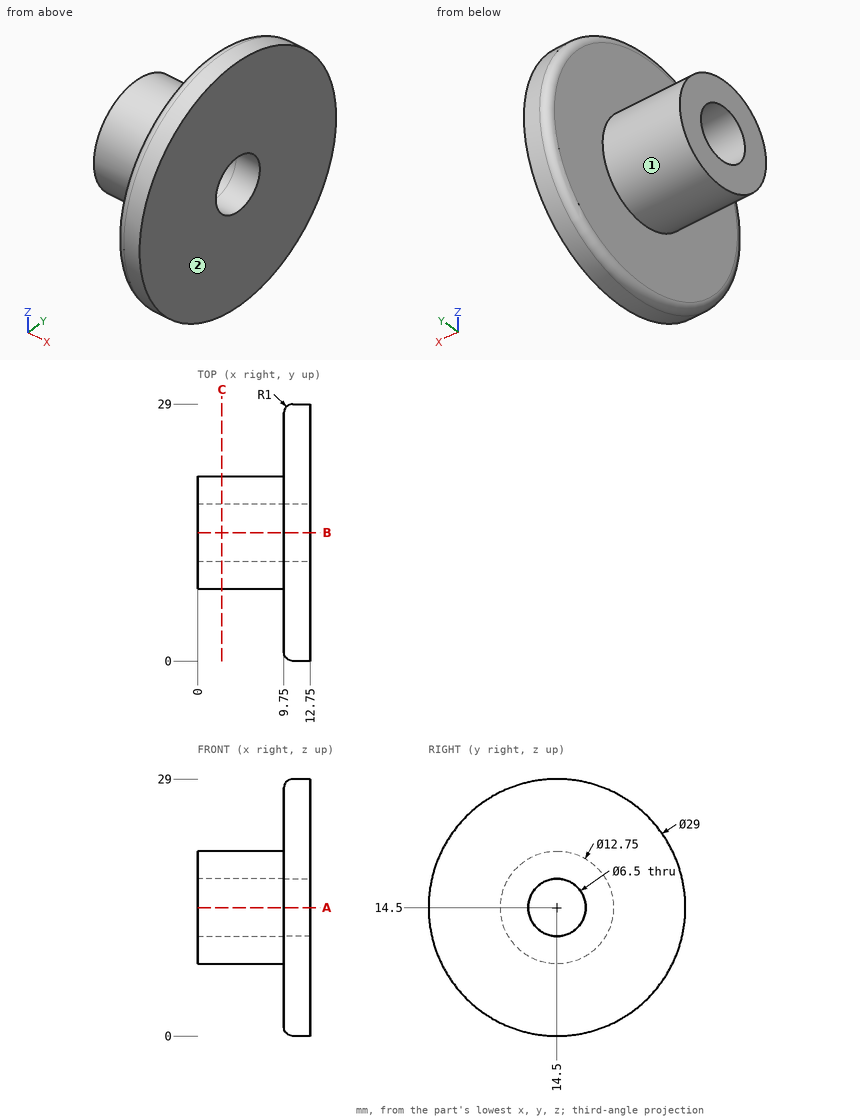
Job drawing, mm, ordinate dimensions from the low corner. One solid piece. A direction names the side the tool comes from. Round coordinates to 2 decimals unless told otherwise and drop trailing zeros. Loops run counter-clockwise (first coordinate to the right, second up) from the corner with the lowest first, then second, coordinate; pieces in that order, holes last. Notation, with made-up numbers: M -34.5,46.25 L 2.5,46.25 A24 cw 2.5,76.25 Z; hole C 54.5,-20.75 d2. An arc over 180 degrees is marked long. One line per question, with ' | ' between items. Start each with the question number.
Item 1: Cut at C-C, the plane x = 2.75. Write the cut outline in (y, z) (3 decimals).
Item 2: Pin check, flat tips, straight feed: pin 1 Ø1 at (x, z) = (8, 10.5) entering from +Y; pin 2 Ø2 at (x, z) = (9, 24) entering from +Y; pin 3 Ø6 at (x, y) = (4, 13) entering from -Z (3 decimals). Stop position of each tip, or through.
Item 3: Cut at A-A, the plane z = 14.5. Write the cut outline in (x, y) (3 decimals).
Item 4: Wall check: line 1 (Y direction, x = 2, z = 14.5) (3 decimals); line 2 (Z direction, x = 10.7, y = 14.5); line 3 (X direction, y = 20.5, z = 12). Give the ranges that are in metal, low to high.
Item 5: Which spindle directions (+Z, -Z, +X, -X, +Y, -Y) get a long thin tool onto all of the face, cutting with end or side? Do the marked faces 1 and 2. Say none if no direction does.
Responses:
1) outline: C 14.5,14.5 d12.75; hole C 14.5,14.5 d6.5
2) pin 1: stops at y = 19.83 | pin 2: stops at y = 25.21 | pin 3: stops at z = 8.125
3) outline: M 0,8.125 L 9.75,8.125 L 9.75,1 A1 ccw 10.75,0 L 12.75,0 L 12.75,11.25 L 0,11.25 Z; M 0,17.75 L 12.75,17.75 L 12.75,29 L 10.75,29 A1 ccw 9.75,28 L 9.75,20.875 L 0,20.875 Z
4) line 1: y = 8.125 to 11.25, 17.75 to 20.875 | line 2: z = 0 to 11.25, 17.75 to 29 | line 3: x = 9.75 to 12.75
5) face 1: -X | face 2: +Z, -Z, +X, +Y, -Y
